The model under review builds one solid part; all positions refer to its coordinate system, in mm. Round coordinates to 2 decimals unless told otherwise and drop trailing zeros. Order: outer loops, then holes, each group sorted by start corner. A loop starts at its lowest first (then second) coordinate and runs counter-clockwise, first axis right, second up. Notation, with made-up numbers: M -4,11 L 15,11 A35 ccw 15,49 Z; hole C 89,24 d8. An arc over 180 degrees is marked long. Answer as a JSON object with one key per item and string values. Group by question number.
1) Insertion check: pin 1 Ø1.2 at (x, z) = (1, 17) entering from -Y; pin 2 Ø1.5 at (x, z) = (1.5, 31) entering from +Y; pin 3 Ø1.2 at (x, y) = (1, 7.5) entering from -Z. Each pin has a flat end and moves straight along its axis. Give the tip position at first contact, or say it passes through.
2) Consider section D-D, the plane y = 19. Write out the cut boundary in (x, z).
3) To check wall thickness, follow line 1 (Y direction, x = 1.7, z = 12.75); line 2 (Y direction, x = 2.6, z = 30); line 3 (Y direction, x = 0.2, z = 31.5). State the ranges of each line that lie inside material, in increasing order.
4) Consider section A-A, the plane z = 12.5. Write out the cut boundary in (x, y), then the cut area to 4 significant figures.
5) Consider section C-C, the plane z = 26.25. Write out the cut boundary in (x, y), then the cut area to 3 significant figures.
```python
from build123d import *

# Parameters (mm, degrees)
F1_DEPTH = 3


with BuildPart() as f1:
    # F0 (on Right) → F1 (new body)
    with BuildSketch(Plane.YZ):
        Polygon((-11.5, 23.945743), (-11.5, 33.945743), (-16.5, 33.945743), (-25, 13.945743), (-25, 10.945743), (0, 10.945743), (0, 13.945743), (8.5, 13.945743), (8.5, 15.945743), (7, 15.945743), (7, 18.445743), (8.5, 18.445743), (8.5, 21.445743), (11.5, 21.445743), (11.5, 18.445743), (13, 18.445743), (13, 15.945743), (11.5, 15.945743), (11.5, 13.945743), (20, 13.945743), (20, 10.945743), (36.5, 10.945743), (36.5, 13.945743), (45, 13.945743), (36.5, 33.945743), (31.5, 33.945743), (31.5, 23.945743), (28.5, 23.945743), (28.5, 33.945743), (-8.5, 33.945743), (-8.5, 23.945743), align=None)
    extrude(amount=F1_DEPTH)


solid = f1.part
```
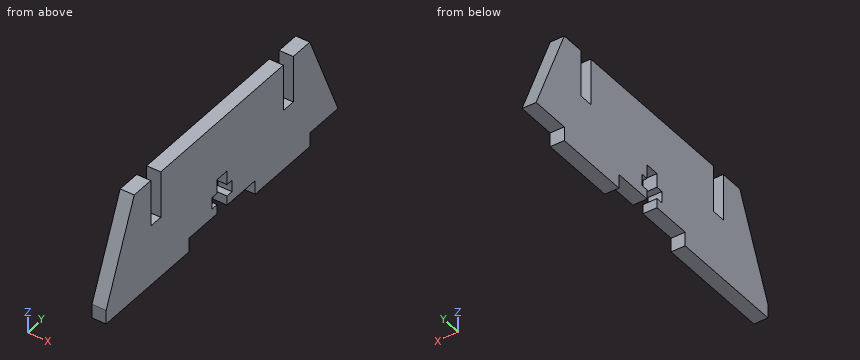
Results list:
{
 "1": {"pin 1": "y = -23.96", "pin 2": "y = 38.07", "pin 3": "z = 13.95"},
 "2": {"outline": "M 0,13.95 L 3,13.95 L 3,33.95 L 0,33.95 Z"},
 "3": {"line 1": "-25 to 0, 20 to 36.5", "line 2": "-18.18 to -11.5, -8.5 to 28.5, 31.5 to 38.18", "line 3": "-17.54 to -11.5, -8.5 to 28.5, 31.5 to 37.54"},
 "4": {"outline": "M 0,-25 L 3,-25 L 3,0 L 0,0 Z; M 0,20 L 3,20 L 3,36.5 L 0,36.5 Z", "area": "124.5 mm^2"},
 "5": {"outline": "M 0,-19.77 L 3,-19.77 L 3,-11.5 L 0,-11.5 Z; M 0,-8.5 L 3,-8.5 L 3,28.5 L 0,28.5 Z; M 0,31.5 L 3,31.5 L 3,39.77 L 0,39.77 Z", "area": "161 mm^2"}
}
